Study the drawing (mm; zero at the part's minimum x, y, z) and answer. A direction names the side the tool comes from. Give positions to 0.01 mm unless a question says otherwise; leave off trailing zeros. Write each loop counter-clockwise with the first axis right and the second up, starting at its lowest first coordinate (ties: lowest second). Pieces come first, ordered by that corner, then holes.
1) Find section A-A (z = 4.25). Determine the outline of the cut face in (x, y).
2) Given pin 1 Ø3 at (x, y) = (25.5, 12) entering from +Z, flat-ended and moving along its own axis, determine where the tip first touches the part or whether it passes through.
3) Find section D-D (y = 7). Determine the outline of the cut face in (x, z).
4) Determine the mould class of the marked faces 1, 2 and 3 for opening direction X: pulls with the +X half, pulls with the -X half, needs draft (parallel to the pull), parting line crosses it, or undercut.
5) Straight lines are drawn through the part: probe 1 along Y at (x, z) = (16, 0.8); probe 2 along Z at (x, y) = (41.45, 2); probe 3 along X at (y, z) = (16, 6.5). For each, find the intervals that lie inside material, in ascending order.
6) A tool of negligible diameter and unlimited length cuts with its end or side. For the marked faces 4 and 5, from which of +Z, -Z, +X, -X, +Y, -Y can it reach the whole face along a straight path? Write none if from no direction.
7) Find section C-C (z = 7). Determine the outline of the cut face in (x, y), plus the area to 3 significant figures.
8) Find section B-B (x = 16). Determine the outline of the cut face in (y, z), plus the area to 3 significant figures.
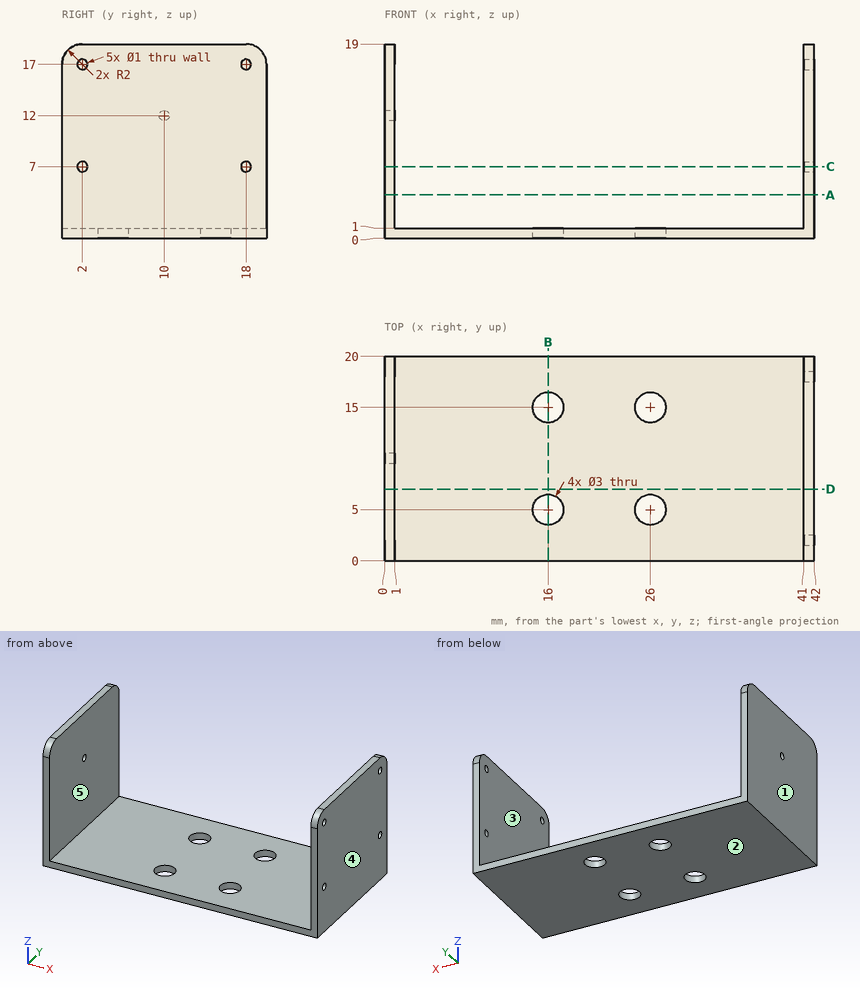
Results:
1. outline: (0, 0) - (1, 0) - (1, 20) - (0, 20) - close; (41, 0) - (42, 0) - (42, 20) - (41, 20) - close
2. pin 1: stops at z = 1
3. outline: (0, 0) - (42, 0) - (42, 19) - (41, 19) - (41, 1) - (1, 1) - (1, 19) - (0, 19) - close
4. face 1: pulls with the -X half
4. face 2: needs draft
4. face 3: undercut
5. probe 1: y = 0 to 3.5, 6.5 to 13.5, 16.5 to 20
5. probe 2: z = 0 to 6.5, 7.5 to 16.5, 17.5 to 19
5. probe 3: x = 0 to 1, 41 to 42
6. face 4: +Z, -Z, +X, +Y, -Y
6. face 5: +Z, +Y, -Y
7. outline: (0, 0) - (1, 0) - (1, 20) - (0, 20) - close; (41, 0) - (42, 0) - (42, 1.5) - (41, 1.5) - close; (41, 2.5) - (42, 2.5) - (42, 17.5) - (41, 17.5) - close; (41, 18.5) - (42, 18.5) - (42, 20) - (41, 20) - close
7. area: 38.0 mm2
8. outline: (0, 0) - (3.5, 0) - (3.5, 1) - (0, 1) - close; (6.5, 0) - (13.5, 0) - (13.5, 1) - (6.5, 1) - close; (16.5, 0) - (20, 0) - (20, 1) - (16.5, 1) - close
8. area: 14.0 mm2
